Part model, mm, in its own coordinate system. Round coordinates to 2 decimals unless told otherwise and drop trailing zeros. Loops run counter-clockwise (first coordinate to the right, second up) from the corner with the lowest first, then second, coordinate; pieces in that order, holes last. Notation, with made-up numbers: M -18.75,-1.75 L -7.75,-1.75 A15 cw -7.75,7.25 Z; hole C -11,61 d4. An arc over 180 degrees is marked long. Answer as CSV lines item,"result". Start each with the question number.
Item 1: Drop flat-ended pins along their axis: pin 1 Ø0.6 at (x, z) = (16.5, 5.5) entering from +Y; pin 2 Ø1 at (y, z) = (-7.5, -114) entering from +X; pin 3 Ø1 at (y, z) = (13.5, -10) entering from +X. Give the stop position or say it passes through.
Item 2: Band-saw the part on B-B (x = 3). Give the cut face in (y, z), and give its area (3 significant figures).
Item 3: Band-saw the part on A-A (y = 0). Give the cut face in (x, z), and give its area (3 significant figures).
Item 4: Band-saw the part on C-C (z = 11). Give the cut face in (x, y), and give its area (3 significant figures).
Item 5: Band-saw the part on D-D (x = -15). Give the cut face in (y, z).
Item 6: Mould opens along X. For faces 1 (the flat face through (6, -19, -150)), 2 (the cylindrical face through (-8.53, 18.48, 4.46)), 3 (the cylindrical face through (-19.28, 0.85, -2.1)), 4 (the cylindrical face through (-20.98, 0.92, 2.1)) say: pulls with the +X half, pulls with the -X half, needs draft (parallel to the pull), parting line crosses it, or undercut.
Item 7: Wall check: line 1 (Y direction, x = 0, z = 78.5); line 2 (Y direction, x = 7.5, z = -64.5); line 3 (X direction, y = 16.5, z = 63). Give the ranges that are in metal, low to high.
```python
from build123d import *

# Parameters (mm, degrees)
F0_R          = 21
F0_R_2        = 19.3
F1_DEPTH      = 150
F3_DEPTH      = 21.001
F4_R          = 10.75
F5_DEPTH      = 21.0010001
F5_DEPTH_BACK = 21.0010001


with BuildPart() as f1:
    # F0 (on Top) → F1 (new body, symmetric)
    with BuildSketch(Plane.XY):
        Circle(F0_R)
        Circle(F0_R_2, mode=Mode.SUBTRACT)
    extrude(amount=F1_DEPTH, both=True)

    # F2 (on Right) → F3 (cut, through all)
    with BuildSketch(Plane.YZ):
        with BuildLine():
            Line((-9, -101), (9, -101))
            ThreePointArc((9, -101), (10.4142135624, -100.4142135624), (11, -99))
            Line((11, -99), (11, 99))
            ThreePointArc((11, 99), (10.4142135624, 100.4142135624), (9, 101))
            Line((9, 101), (-9, 101))
            ThreePointArc((-9, 101), (-10.4142135624, 100.4142135624), (-11, 99))
            Line((-11, 99), (-11, -99))
            ThreePointArc((-11, -99), (-10.4142135624, -100.4142135624), (-9, -101))
        make_face()
    extrude(amount=F3_DEPTH, mode=Mode.SUBTRACT)

    # F4 (on Front) → F5 (cut, two sides)
    with BuildSketch(Plane.XZ) as f5_sk:
        with Locations((0, 11)):
            Circle(F4_R)
    extrude(amount=-F5_DEPTH, mode=Mode.SUBTRACT)
    extrude(f5_sk.sketch, amount=F5_DEPTH_BACK, mode=Mode.SUBTRACT)


solid = f1.part
```
Answer block:
1,pin 1,"stops at y = 13.36"
1,pin 2,"stops at x = 19.8"
1,pin 3,"stops at x = 16.49"
2,outline,"M -20.78,-150 L -19.07,-150 L -19.07,0.68 L -20.78,0.68 Z; M -20.78,21.32 L -19.07,21.32 L -19.07,150 L -20.78,150 Z; M 19.07,-150 L 20.78,-150 L 20.78,0.68 L 19.07,0.68 Z; M 19.07,21.32 L 20.78,21.32 L 20.78,150 L 19.07,150 Z"
2,area,"961 mm^2"
3,outline,"M -21,-150 L -19.3,-150 L -19.3,150 L -21,150 Z; M 19.3,-150 L 21,-150 L 21,-101 L 19.3,-101 Z; M 19.3,101 L 21,101 L 21,150 L 19.3,150 Z"
3,area,"677 mm^2"
4,outline,"M -10.75,-18.04 L -10.75,-16.03 A19.3 cw -10.75,16.03 L -10.75,18.04 A21 ccw Z; M 10.75,-18.04 A21 ccw 17.89,-11 L 15.86,-11 A19.3 cw 10.75,-16.03 Z; M 10.75,16.03 A19.3 cw 15.86,11 L 17.89,11 A21 ccw 10.75,18.04 Z"
4,area,"98.5 mm^2"
5,outline,"M -14.7,-150 L -12.14,-150 L -12.14,150 L -14.7,150 Z; M 12.14,-150 L 14.7,-150 L 14.7,150 L 12.14,150 Z"
6,face 1,"needs draft"
6,face 2,"undercut"
6,face 3,"undercut"
6,face 4,"parting line crosses it"
7,line 1,"y = -21 to -19.3, 19.3 to 21"
7,line 2,"y = -19.62 to -17.78, 17.78 to 19.62"
7,line 3,"x = -12.99 to -10.01, 10.01 to 12.99"
